Work out the finished part from the listing and answer in its coordinate system (mm). Round coordinates to 2 decimals unless told otherwise and drop trailing zeros. Write each loop counter-clockwise with the first axis right and the second up, starting at its lowest first coordinate (ties: lowest second). Pieces come first, ordered by that corner, then holes. Notation, with made-up numbers: (75.25, 10) - (114.25, 10) arc R16 cw to (114.25, 40) - close; hole circle Ø2 at (-9, 26). An arc over 180 degrees is marked (long way). Answer as a JSON object with one key per item and string values.
```python
from build123d import *

# Parameters (mm, degrees)
F1_DEPTH = 1524
F2_R     = 1.27


with BuildPart() as f1:
    # F0 (on Front) → F1 (new body)
    with BuildSketch(Plane.XZ):
        with BuildLine():
            ThreePointArc((-45.3183636102, -3.556), (-44.243239134, -1.9205395258), (-43.8662092519, 0))
            Line((-43.8662092519, 0), (-48.9462092519, 0))
            Line((-48.9462092519, 0), (-48.9462092519, -3.556))
            Line((-48.9462092519, -3.556), (-45.3183636102, -3.556))
        make_face()
        with BuildLine():
            Line((-48.9462092519, 0), (-43.8662092519, 0))
            ThreePointArc((-43.8662092519, 0), (-45.3541068035, 3.5921024484), (-48.9462092519, 5.08))
            Line((-48.9462092519, 5.08), (-48.9462092519, 0))
        make_face()
        with BuildLine():
            ThreePointArc((-48.9462092519, -5.08), (-46.978733712, -4.6835285843), (-45.3183636102, -3.556))
            Line((-45.3183636102, -3.556), (-48.9462092519, -3.556))
            Line((-48.9462092519, -3.556), (-48.9462092519, -5.08))
        make_face()
        with BuildLine():
            Line((-48.9462092519, 0), (-48.9462092519, 5.08))
            ThreePointArc((-48.9462092519, 5.08), (-54.0262092519, 0), (-48.9462092519, -5.08))
            Line((-48.9462092519, -5.08), (-48.9462092519, -3.556))
            Line((-48.9462092519, -3.556), (-48.9462092519, 0))
        make_face()
        with BuildLine():
            Line((-12.3658548936, -3.556), (-45.3183636102, -3.556))
            ThreePointArc((-45.3183636102, -3.556), (-46.978733712, -4.6835285843), (-48.9462092519, -5.08))
            Line((-48.9462092519, -5.08), (-48.9462092519, -8.89))
            Line((-48.9462092519, -8.89), (-8.7380092519, -8.89))
            Line((-8.7380092519, -8.89), (-8.7380092519, -5.08))
            ThreePointArc((-8.7380092519, -5.08), (-10.7054847918, -4.6835285843), (-12.3658548936, -3.556))
        make_face()
        with BuildLine():
            Line((-8.7380092519, 0), (-13.8180092519, 0))
            ThreePointArc((-13.8180092519, 0), (-13.4409793698, -1.9205395258), (-12.3658548936, -3.556))
            Line((-12.3658548936, -3.556), (-8.7380092519, -3.556))
            Line((-8.7380092519, -3.556), (-8.7380092519, 0))
        make_face()
        with BuildLine():
            ThreePointArc((-8.7380092519, 5.08), (-12.3301117003, 3.5921024484), (-13.8180092519, 0))
            Line((-13.8180092519, 0), (-8.7380092519, 0))
            Line((-8.7380092519, 0), (-8.7380092519, 5.08))
        make_face()
        with BuildLine():
            Line((-8.7380092519, -3.556), (-12.3658548936, -3.556))
            ThreePointArc((-12.3658548936, -3.556), (-10.7054847918, -4.6835285843), (-8.7380092519, -5.08))
            Line((-8.7380092519, -5.08), (-8.7380092519, -3.556))
        make_face()
        with BuildLine():
            Line((-8.7380092519, 5.08), (-8.7380092519, 0))
            Line((-8.7380092519, 0), (-8.7380092519, -3.556))
            Line((-8.7380092519, -3.556), (-8.7380092519, -5.08))
            ThreePointArc((-8.7380092519, -5.08), (-5.1459068035, -3.5921024484), (-3.6580092519, 0))
            ThreePointArc((-3.6580092519, 0), (-5.1459068035, 3.5921024484), (-8.7380092519, 5.08))
        make_face()
    extrude(amount=F1_DEPTH)

    # F2
    f2_edges = [f1.edges().sort_by_distance(p)[0] for p in [
        (-45.318364, -762, -3.556),
        (-12.365855, -762, -3.556),
    ]]
    fillet(f2_edges, radius=F2_R)


solid = f1.part
```
Item 1: Consider line 1 along Z through (x, y) = (-20, -882.5); line 2 along X through (y, z) = (-290, -1); line 3 along X through (y, z) = (-596.5, 4). Determine where each line is inside the solid, lowest interval first.
Results found:
{"line 1": "-8.89 to -3.56", "line 2": "-53.93 to -43.97, -13.72 to -3.76", "line 3": "-52.08 to -45.81, -11.87 to -5.61"}
Item 2: A cutting plane is placed at A-A (y = -1252.5). Write down the section's boundary in (x, z).
Results found:
{"outline": "(-48.95, -8.89) - (-8.74, -8.89) - (-8.74, -5.08) arc R5.08 ccw (long way) to (-13.48, -1.83) arc R1.27 cw to (-14.66, -3.56) - (-43.02, -3.56) arc R1.27 cw to (-44.21, -1.83) arc R5.08 ccw (long way) to (-48.95, -5.08) - close"}
Item 3: Each of these flat-tipped pins is pushed along its axis until it touches: P1, Ø5, axis at y = -339.5, z = -4, coming from the +X side; P2, Ø5, axis at y = -926.5, z = -1, coming from the +X side; P3, Ø1.1, axis at y = -590, z = -7, coming from the +X side; P4, Ø4, axis at y = -382, z = -7.5, coming from the -X side. Where does it stop, or does it pass through?
Results found:
{"P1": "x = -3.88", "P2": "x = -3.66", "P3": "x = -8.74", "P4": "x = -48.95"}
Item 4: Determine the mould class of faces 1 (the flat face through (-29, -751, -3.556)), 2 (the flat face through (-29, -751, -8.89)) for opening direction X: pulls with the +X half, pulls with the -X half, needs draft (parallel to the pull), parting line crosses it, or undercut.
Results found:
{"face 1": "undercut", "face 2": "needs draft"}
